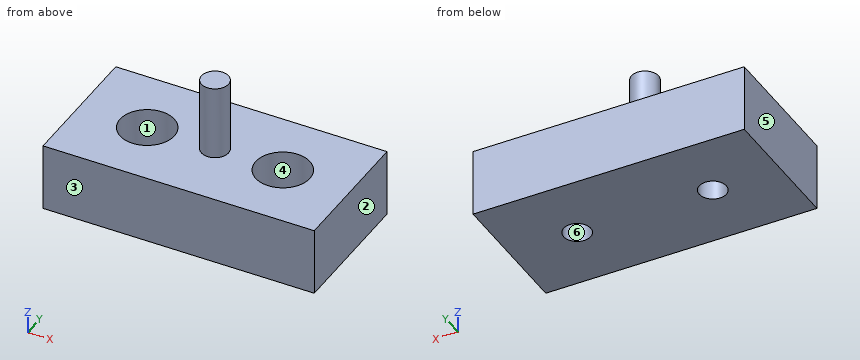
from build123d import *

# Parameters (mm, degrees)
SKETCH_1_W          = 20
SKETCH_1_H          = 10
SKETCH_1_R          = 1
EXTRUDE_1_DEPTH     = 5
SKETCH_2_R          = 1
EXTRUDE_2_DEPTH     = 5.5
SKETCH_4_R          = 2
CUT_EXTRUDE_2_DEPTH = 3


with BuildPart() as part:
    # 草图1 → 凸台-拉伸1 (new body)
    with BuildSketch(Plane.XY):
        Rectangle(SKETCH_1_W, SKETCH_1_H)
        with Locations((-5, 0)):
            Circle(SKETCH_1_R, mode=Mode.SUBTRACT)
        with Locations((5, 0)):
            Circle(SKETCH_1_R, mode=Mode.SUBTRACT)
    extrude(amount=EXTRUDE_1_DEPTH)

    # 草图2 → 凸台-拉伸2 (add)
    with BuildSketch(Plane.XY.offset(5)):
        Circle(SKETCH_2_R)
    extrude(amount=EXTRUDE_2_DEPTH)

    # 草图4 → 切除-拉伸2 (cut)
    with BuildSketch(Plane.XY.offset(5)):
        with Locations((5, 0)):
            Circle(SKETCH_4_R)
        with Locations((-5, 0)):
            Circle(SKETCH_4_R)
    extrude(amount=-CUT_EXTRUDE_2_DEPTH, mode=Mode.SUBTRACT)


solid = part.part
Source: CAD feature listing. Evaluate the final solid. Frame: model axes, mm. Face numbers are marked on the shaded views. A direction names the side the tool comes from. Coordinates: 2 decimals unless noted, no trailing zeros. Order: outer loops, then holes, each group sorted by start corner. A loop starts at its lowest first (then second) coordinate and runs counter-clockwise, first axis right, second up. Notation, with made-up numbers: M 60,80.25 L 96,80.25 A22 ccw 96,114.25 Z; hole C 14,-19 d7. An arc over 180 degrees is marked long. Write each question's results on one line, items separated by ' | '. Start each with the question number.
1. Section C-C, the plane z = 0.75. Return the cut outline in (x, y).
2. Section D-D, the plane x = 0. Return the cut outline in (y, z).
3. Pin query (flat end, axial travel): pin 1 (4 mm diameter, centred on x = 0.5, y = 3.5, fed in from +Z). Return the tip coordinate at first contact, or that it passes through.
4. Reachability of the marked faces 1 and 2 from +Z, -Z, +X, -X, +Y, -Y: full face, straight path, thin tool, end or side. Return the list, or none.
5. Section A-A, the plane y = 0. Return the cut outline in (x, z), then the cut area to 3 significant figures.
6. Material intervals for L1, parallel to X at y = 0, z = 0.5; L2, parallel to Y at x = -5, z = 1.2; L3, parallel to Y at x = -5, z = 3.4, sorted ascending.
7. Draft query along Y for the marked faces 3, 4, 5 and 6. Return one class per face: +Y half, -Y half, draft (parallel to the pull), parting line (faces both ways), or undercut.
8. Section B-B, the plane x = 5. Return the cut outline in (y, z), then the cut area to 3 significant figures.
Solution:
1) outline: M -10,-5 L 10,-5 L 10,5 L -10,5 Z; hole C -5,0 d2; hole C 5,0 d2
2) outline: M -5,0 L 5,0 L 5,5 L 1,5 L 1,10.5 L -1,10.5 L -1,5 L -5,5 Z
3) pin 1: z = 5
4) face 1: +Z | face 2: +Z, -Z, +X, +Y, -Y
5) outline: M -10,0 L -6,0 L -6,2 L -7,2 L -7,5 L -10,5 Z; M -4,0 L 4,0 L 4,2 L 3,2 L 3,5 L 1,5 L 1,10.5 L -1,10.5 L -1,5 L -3,5 L -3,2 L -4,2 Z; M 6,0 L 10,0 L 10,5 L 7,5 L 7,2 L 6,2 Z | area: 79.0 mm²
6) L1: -10 to -6, -4 to 4, 6 to 10 | L2: -5 to -1, 1 to 5 | L3: -5 to -2, 2 to 5
7) face 3: -Y half | face 4: undercut | face 5: draft | face 6: undercut
8) outline: M -5,0 L -1,0 L -1,2 L -2,2 L -2,5 L -5,5 Z; M 1,0 L 5,0 L 5,5 L 2,5 L 2,2 L 1,2 Z | area: 34.0 mm²
